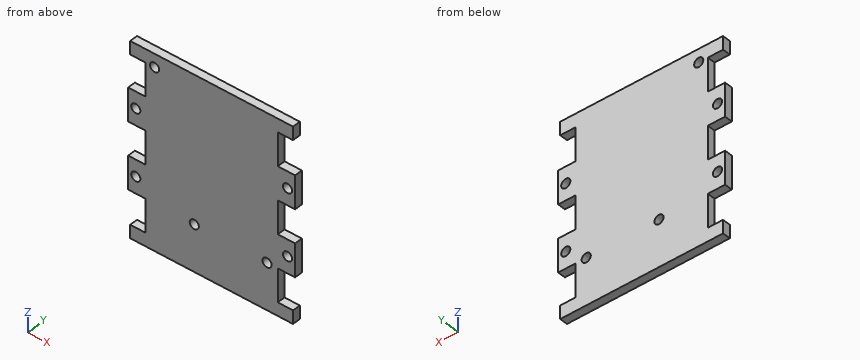
from build123d import *

# Parameters (mm, degrees)
SKETCH1_R           = 1.7526
BOSS_EXTRUDE1_DEPTH = 3.048
SKETCH2_R           = 1.7526
CUT_EXTRUDE1_DEPTH  = 49.908368221


with BuildPart() as part:
    # Sketch1 → Boss-Extrude1 (new body)
    with BuildSketch(Plane(origin=(0, 0, 0), x_dir=(1, 0, 0), z_dir=(0, 1, 0))):
        Polygon((31.242, -36.83), (-31.242, -36.83), (-31.242, -31.75), (-25.4, -31.75), (-25.4, -19.05), (-31.242, -19.05), (-32.03575, -19.05), (-32.03575, -6.35), (-31.242, -6.35), (-25.4, -6.35), (-25.4, 6.35), (-31.242, 6.35), (-32.03575, 6.35), (-32.03575, 19.05), (-31.242, 19.05), (-25.4, 19.05), (-25.4, 31.75), (-31.242, 31.75), (-31.242, 36.83), (31.242, 36.83), (31.242, 31.75), (25.4, 31.75), (25.4, 19.05), (31.242, 19.05), (32.03575, 19.05), (32.03575, 6.35), (31.242, 6.35), (25.4, 6.35), (25.4, -6.35), (31.242, -6.35), (32.03575, -6.35), (32.03575, -19.05), (31.242, -19.05), (25.4, -19.05), (25.4, -31.75), (31.242, -31.75), align=None)
        with Locations(Location((-29.11475, 12.7, 0), (0, 0, 90))):
            Circle(SKETCH1_R, mode=Mode.SUBTRACT)
        with Locations(Location((-29.11475, -12.7, 0), (0, 0, 90))):
            Circle(SKETCH1_R, mode=Mode.SUBTRACT)
        with Locations(Location((29.11475, -12.7, 0), (0, 0, 90))):
            Circle(SKETCH1_R, mode=Mode.SUBTRACT)
        with Locations(Location((29.11475, 12.7, 0), (0, 0, 90))):
            Circle(SKETCH1_R, mode=Mode.SUBTRACT)
    extrude(amount=BOSS_EXTRUDE1_DEPTH)

    # Sketch2 → Cut-Extrude1 (cut, through all)
    with BuildSketch(Plane(origin=(0, 3.048, 0), x_dir=(1, 0, 0), z_dir=(0, 1, 0))):
        with Locations(Location((21.2725, 19.05, 0), (0, 0, 270))):
            Circle(SKETCH2_R)
        with Locations(Location((-6.6675, 19.05, 0), (0, 0, 270))):
            Circle(SKETCH2_R)
        with Locations(Location((-21.9075, -31.75, 0), (0, 0, 270))):
            Circle(SKETCH2_R)
    extrude(amount=-CUT_EXTRUDE1_DEPTH, mode=Mode.SUBTRACT)


solid = part.part
Geometry: final body of the model. Coordinates: model frame, mm. Coordinates: 2 decimals unless noted, no trailing zeros. Loops run counter-clockwise (first coordinate to the right, second up) from the corner with the lowest first, then second, coordinate; pieces in that order, holes last. Notation, with made-up numbers: (35, -20.5) - (87, -20.5) arc R23 ccw to (87, -11.5) - close; hole circle Ø8 at (-33.5, 52). An arc over 180 degrees is marked (long way). One line per question, with ' | ' between items. Start each with the question number.
(1) Ray query, L1, parallel to Z at x = -27, y = 1.4; L2, parallel to X at y = 0.9, z = -12.7; L3, parallel to X at y = 1.85, z = 31.5. Return the intervals inside material, ascending. Write a range as from..to.
(2) First-contact query: pin 1 (1 mm diameter, centred on y = 2, z = -4, fed in from -X); pin 2 (4.5 mm diameter, centred on x = 29.11, z = 12.7, fed in from +Y); pin 3 (1.5 mm diameter, centred on y = 1.5, z = 33.5, fed in from +X); pin 4 (0.9 mm diameter, centred on y = 1, z = -2, fed in from +X). Flat tips, straight axial feed; report the tip coordinate or a pass-through.
(3) Cut plane B-B on y = 1.9. Count the separate pieces of the cut face and the enclosed holes in it, and give its area (3 significant figures).
(4) Cut plane A-A on z = -12.7. Output: boundary loops of the cut face in (x, y).
(5) Cut plane C-C on z = 26. Output: boundary loops of the cut face in (x, y).
Here are the results:
1) L1: -36.83..-31.75, -19.05..-6.35, 6.35..19.05, 31.75..36.83 | L2: -32.04..-30.87, -27.36..27.36, 30.87..32.04 | L3: -25.4..-23.64, -20.17..25.4
2) pin 1: x = -25.4 | pin 2: y = 3.05 | pin 3: x = 31.24 | pin 4: x = 25.4
3) separate pieces: 1 | enclosed holes: 7 | area: 4,130 mm²
4) outline: (-32.04, 0) - (-30.87, 0) - (-30.87, 3.05) - (-32.04, 3.05) - close; (-27.36, 0) - (27.36, 0) - (27.36, 3.05) - (-27.36, 3.05) - close; (30.87, 0) - (32.04, 0) - (32.04, 3.05) - (30.87, 3.05) - close
5) outline: (-25.4, 0) - (25.4, 0) - (25.4, 3.05) - (-25.4, 3.05) - close
